Verification items for the finished model (mm, model axes). A direction names the side the tool comes from. Give positions to 0.01 mm unless a question says otherwise; leave off trailing zeros. Order: outer loops, then holes, each group sorted by start corner. A loop starts at its lowest first (then second) coordinate and runs counter-clockwise, first axis right, second up. Notation, with made-up numbers: (0.25, -5) -> (42.25, -5) arc R26 cw to (42.25, 24) -> close; hole circle Ø9 at (3, 38.5). An arc over 180 degrees is marked (long way). Return JSON: item names as keys, results as strings. Group by question number.
(1) Release check for a two-part mould opening along X. For faces 1 (the face through (10, 11, -8)), 2 (the face through (2, 10, -2.15)), 3 (the face through (14.765, -1.288, 0.035)) record: pulls with the +X half, pulls with the -X half, needs draft (parallel to the pull), parting line crosses it, or undercut.
(2) Thickness scan on line 1 along Z through (x, y) = (8.75, 3.25); line 2 along Z through (x, y) = (6.5, 1.75); line 3 along X through (y, z) = (11.25, -6.25). Record the ranges inside material, lowest first.
(3) Tool access check on faces 4 (the face through (-1, 15, 2.5)), 5 (the face through (3, 11, 3)), 6 (the face through (2, -1, 2.5)). Record the directions out of +Z, -Z, +X, -X, +Y, -Y that give a thin tool (end or side, any length) a straight path to the whole face; none if there is none.
(4) Cross-section at D-D on z = -5. Enter the section's corners in (x, y), then the cut area to 3 significant figures.
(5) Cross-section at A-A on y = 13.25. Enter the section's corners in (x, z), then the cut area to 4 significant figures.
(6) Depth check by flat-ended pin: pin 1 Ø0.9 at (x, y) = (15, -0.5) entering from -Z; pin 2 Ø1.5 at (y, z) = (4, -2.5) entering from +X; pin 3 Ø0.9 at (x, y) = (2.5, -0.5) entering from +Z. Enter the tip coordinate at first touch or a pass-through.
(7) Cross-section at B-B on x = 9.5. Enter the section's corners in (y, z).
(8) Cross-section at C-C on z = 0. State how many separate pieces and enclosed holes the cut face has, then the cut area to 3 significant figures.
from build123d import *

# Parameters (mm, degrees)
BOSS_EXTRUDE1_DEPTH = 9
CUT_EXTRUDE1_DEPTH  = 7.5
CUT_EXTRUDE2_DEPTH  = 2.15
BOSS_EXTRUDE2_DEPTH = 2.5


with BuildPart() as part:
    # Sketch1 → Boss-Extrude1 (new body, symmetric)
    with BuildSketch(Plane.XY):
        Polygon((0, 0), (0, 18), (3, 18), (18, 3), (18, 0), align=None)
    extrude(amount=BOSS_EXTRUDE1_DEPTH, both=True)

    # Sketch2 → Cut-Extrude1 (cut, symmetric)
    with BuildSketch(Plane.XY):
        Polygon((3, 18), (3, 3), (18, 3), align=None)
    extrude(amount=CUT_EXTRUDE1_DEPTH, both=True, mode=Mode.SUBTRACT)

    # Sketch3 → Cut-Extrude2 (cut, symmetric)
    with BuildSketch(Plane.XY):
        Polygon((0, 14), (3, 14), (3, 7), (0, 4), align=None)
        Polygon((7, 3), (14, 3), (14, 0), (4, 0), align=None)
    extrude(amount=CUT_EXTRUDE2_DEPTH, both=True, mode=Mode.SUBTRACT)

    # Sketch4 → Boss-Extrude2 (add, symmetric)
    with BuildSketch(Plane.XY):
        Polygon((1.504575227, -1.8), (0.511249685, -0.790946088), (1.234750477, 0), (3.535533906, 0), align=None)
        Polygon((0, 3.535533906), (-1.8, 1.504575227), (-0.790946088, 0.511249685), (0, 1.234750477), align=None)
        Polygon((0, 17.3), (0, 14.999216572), (-0.790946088, 14.275715779), (-1.8, 15.269041321), align=None)
        Polygon((14.999216572, 0), (14.275715779, -0.790946088), (15.269041321, -1.8), (17.3, 0), align=None)
    extrude(amount=BOSS_EXTRUDE2_DEPTH, both=True)


solid = part.part
Verdict:
{
 "1": {"face 1": "pulls with the +X half", "face 2": "needs draft", "face 3": "undercut"},
 "2": {"line 1": "-9 to -7.5, 7.5 to 9", "line 2": "-9 to -2.15, 2.15 to 9", "line 3": "0 to 3"},
 "3": {"face 4": "+Z, -X, +Y, -Y", "face 5": "+X, +Y", "face 6": "+Z, +X, -X, -Y"},
 "4": {"outline": "(0, 0) -> (18, 0) -> (18, 3) -> (3, 3) -> (3, 18) -> (0, 18) -> close", "area": "99.0 mm²"},
 "5": {"outline": "(0, -9) -> (7.75, -9) -> (7.75, -7.5) -> (3, -7.5) -> (3, -2.15) -> (0, -2.15) -> close; (0, 2.15) -> (3, 2.15) -> (3, 7.5) -> (7.75, 7.5) -> (7.75, 9) -> (0, 9) -> close", "area": "55.35 mm²"},
 "6": {"pin 1": "z = -2.5", "pin 2": "x = 3", "pin 3": "z = 2.5"},
 "7": {"outline": "(0, -9) -> (11.5, -9) -> (11.5, -7.5) -> (3, -7.5) -> (3, -2.15) -> (0, -2.15) -> close; (0, 2.15) -> (3, 2.15) -> (3, 7.5) -> (11.5, 7.5) -> (11.5, 9) -> (0, 9) -> close"},
 "8": {"separate pieces": "3", "enclosed holes": "0", "area": "59.3 mm²"}
}
